The model under review builds one solid part; all positions refer to its coordinate system, in mm. Coordinates: 2 decimals unless noted, no trailing zeros. Use one line per item in the form item = value. Start each with the question number.
(1) Insertion check: pin 1 Ø3 at (x, z) = (-0.22, 1.97) entering from +Y. The pin has a flat end and moves straight along its axis. Give the tip position at first contact, or say it passes through.
(2) Wall thickness on line 1 along Z through (x, y) = (21.5, 1.3); line 2 along Z through (x, y) = (26, 0.4): over which ranges is each line inside the solid? List them lowest first.
(3) Mouldability with a two-part tool opening along X and no side actions: class faces 1 (the cylindrical face through (-28.72, 0.99, 30.54)), 2 (the cylindrical face through (22.957, 1.014, 9.234)), 3 (the flat face through (29.781, 1, 2)) as +X half, -X half, draft (parallel to the pull), parting line (faces both ways), or undercut.
```python
from build123d import *

# Parameters (mm, degrees)
BOSS_EXTRUDE1_DEPTH = 2
SKETCH2_R           = 1
CUT_EXTRUDE1_DEPTH  = 3


with BuildPart() as part:
    # Sketch1 → Boss-Extrude1 (new body)
    with BuildSketch(Plane(origin=(0, 0, 0), x_dir=(1, 0, 0), z_dir=(0, 1, 0))):
        with BuildLine():
            Line((-25.218978102, 28.02919708), (24.781021898, 28.02919708))
            ThreePointArc((24.781021898, 28.02919708), (28.316555804, 26.564730986), (29.781021898, 23.02919708))
            Line((29.781021898, 23.02919708), (29.781021898, -26.97080292))
            ThreePointArc((29.781021898, -26.97080292), (28.316555804, -30.506336826), (24.781021898, -31.97080292))
            Line((24.781021898, -31.97080292), (-25.218978102, -31.97080292))
            ThreePointArc((-25.218978102, -31.97080292), (-28.754512008, -30.506336826), (-30.218978102, -26.97080292))
            Line((-30.218978102, -26.97080292), (-30.218978102, 23.02919708))
            ThreePointArc((-30.218978102, 23.02919708), (-28.754512008, 26.564730986), (-25.218978102, 28.02919708))
        make_face()
    extrude(amount=BOSS_EXTRUDE1_DEPTH)

    # Sketch2 → Cut-Extrude1 (cut)
    with BuildSketch(Plane(origin=(0, 2, 0), x_dir=(1, 0, 0), z_dir=(0, 1, 0))):
        with Locations(Location((-22.718978102, 6.02919708, 0), (0, 0, 270))):
            Circle(SKETCH2_R)
        with Locations(Location((-22.718978102, -9.97080292, 0), (0, 0, 270))):
            Circle(SKETCH2_R)
        with Locations(Location((22.281021898, 5.669895239, 0), (0, 0, 270))):
            Circle(SKETCH2_R)
        with Locations(Location((22.281021898, -9.97080292, 0), (0, 0, 270))):
            Circle(SKETCH2_R)
        with Locations(Location((-0.218978102, -1.97080292, 0), (0, 0, 270))):
            Circle(SKETCH2_R)
    extrude(amount=-CUT_EXTRUDE1_DEPTH, mode=Mode.SUBTRACT)


solid = part.part
```
Findings:
q1.pin_1 = 2
q2.line_1 = -28.03 to -6.29, -5.05 to 9.35, 10.6 to 31.97
q2.line_2 = -27.88 to 31.82
q3.face_1 = -X half
q3.face_2 = undercut
q3.face_3 = +X half
